from build123d import *

# Parameters (mm, degrees)
EXTRUDE_1_DEPTH      = 5
SKETCH_2_R           = 4
CUT_EXTRUDE_1_DEPTH  = 5
SKETCH_3_R           = 7.5
CUT_EXTRUDE_2_DEPTH  = 10
CUT_EXTRUDE_START    = -10
CUT_EXTRUDE_3_DEPTH  = 10
CUT_EXTRUDE_4_DEPTH  = 10
FILLET_1_R           = 2
SKETCH_6_R           = 6.525
CUT_EXTRUDE_5_DEPTH  = 10
SKETCH_8_R           = 1.5
CUT_EXTRUDE_7_DEPTH  = 10
SKETCH_11_R          = 0.8
CUT_EXTRUDE_8_DEPTH  = 10
SKETCH_13_R          = 1.65
EXTRUDE_3_DEPTH      = 5
FILLET_3_R           = 10
CUT_EXTRUDE_9_DEPTH  = 5
SKETCH_16_W          = 48
SKETCH_16_H          = 16
SKETCH_16_W_2        = 50
CUT_EXTRUDE_10_DEPTH = 2
FILLET_4_SIZE        = 8
SKETCH_17_R          = 12.5
SKETCH_17_R_2        = 12.25
CUT_EXTRUDE_11_DEPTH = 1


with BuildPart() as part:
    # 草图1 → 凸台-拉伸1 (new body)
    with BuildSketch(Plane.XY):
        with BuildLine():
            Line((-30.736828822, 22.472146181), (-0.685809887, 14.645629979))
            ThreePointArc((-0.685809887, 14.645629979), (1.813935823, 14.162064114), (4.35486081, 14))
            Line((4.35486081, 14), (116.18070798, 14))
            ThreePointArc((116.18070798, 14), (120.501201779, 14.472241979), (124.617663724, 15.866666667))
            ThreePointArc((124.617663724, 15.866666667), (149.5, 0), (124.617663724, -15.866666667))
            ThreePointArc((124.617663724, -15.866666667), (120.501201779, -14.472241979), (116.18070798, -14))
            Line((116.18070798, -14), (0, -14))
            ThreePointArc((0, -14), (-4.256709716, -13.337181951), (-8.110358856, -11.411488914))
            Line((-8.110358856, -11.411488914), (-36.971915435, 9.10095979))
            ThreePointArc((-36.971915435, 9.10095979), (-39.424388736, 18.383894386), (-30.736828822, 22.472146181))
        make_face()
    extrude(amount=EXTRUDE_1_DEPTH)

    # 草图2 → 切除-拉伸1 (cut)
    with BuildSketch(Plane.XY.offset(5)):
        with Locations((-32.627080333, 15.214257423)):
            Circle(SKETCH_2_R)
    extrude(amount=-CUT_EXTRUDE_1_DEPTH, mode=Mode.SUBTRACT)

    # 草图3 → 切除-拉伸2 (cut)
    with BuildSketch(Plane.XY.offset(5)):
        Circle(SKETCH_3_R)
    extrude(amount=-CUT_EXTRUDE_2_DEPTH, mode=Mode.SUBTRACT)

    # 草图4 → 切除-拉伸3 (cut)
    with BuildSketch(Plane.XY.offset(5).offset(CUT_EXTRUDE_START)):
        with BuildLine():
            ThreePointArc((-13.498186757, -0.221256097), (-12.235155125, 5.705346533), (-8.506975197, 10.482431635))
            Line((-8.506975197, 10.482431635), (-25.137780404, 14.813774499))
            ThreePointArc((-25.137780404, 14.813774499), (-25.829771931, 12.04462046), (-27.506263415, 9.73454629))
            Line((-27.506263415, 9.73454629), (-13.498186757, -0.221256097))
        make_face()
    extrude(amount=CUT_EXTRUDE_3_DEPTH, mode=Mode.SUBTRACT)

    # 草图5 → 切除-拉伸4 (cut)
    with BuildSketch(Plane.XY.offset(5).offset(CUT_EXTRUDE_START)):
        Polygon((33.945349397, 8), (17.945349397, -8), (33.945349397, -8), align=None)
        with BuildLine():
            ThreePointArc((13.5, 0), (12.826784504, -4.209940534), (10.874281585, -8))
            Line((10.874281585, -8), (26.874281585, 8))
            Line((26.874281585, 8), (10.874281585, 8))
            ThreePointArc((10.874281585, 8), (12.826784504, 4.209940534), (13.5, 0))
        make_face()
        Polygon((54.945349397, -8), (38.945349397, 8), (38.945349397, -8), align=None)
        Polygon((62.016417209, 8), (46.016417209, 8), (62.016417209, -8), align=None)
        Polygon((83.016417209, 8), (67.016417209, 8), (67.016417209, -8), align=None)
        Polygon((90.087485021, 8), (74.087485021, -8), (90.087485021, -8), align=None)
    extrude(amount=CUT_EXTRUDE_4_DEPTH, mode=Mode.SUBTRACT)

    # 圆角1
    fillet_1_edges = [part.edges().sort_by_distance(p)[0] for p in [
        (38.945349397, 8, 2.5),
        (54.945349397, -8, 2.5),
        (38.945349397, -8, 2.5),
        (10.874281585, -8, 2.5),
        (10.874281585, 8, 2.5),
        (26.874281585, 8, 2.5),
        (90.087485021, 8, 2.5),
        (90.087485021, -8, 2.5),
        (74.087485021, -8, 2.5),
        (17.945349397, -8, 2.5),
        (33.945349397, 8, 2.5),
        (33.945349397, -8, 2.5),
        (-27.506263415, 9.73454629, 2.5),
        (-25.137780404, 14.813774499, 2.5),
        (-8.506975197, 10.482431635, 2.5),
        (-13.498186757, -0.221256097, 2.5),
        (67.016417209, -8, 2.5),
        (67.016417209, 8, 2.5),
        (83.016417209, 8, 2.5),
        (62.016417209, -8, 2.5),
        (46.016417209, 8, 2.5),
        (62.016417209, 8, 2.5),
    ]]
    fillet(fillet_1_edges, radius=FILLET_1_R)

    # 草图6 → 切除-拉伸5 (cut)
    with BuildSketch(Plane.XY.offset(5)):
        with Locations((132, 0)):
            Circle(SKETCH_6_R)
    extrude(amount=-CUT_EXTRUDE_5_DEPTH, mode=Mode.SUBTRACT)

    # 草图8 → 切除-拉伸7 (cut)
    with BuildSketch(Plane.XY.offset(5)):
        with Locations((141.5, 0)):
            Circle(SKETCH_8_R)
        with Locations((127.25, -8.227241336)):
            Circle(SKETCH_8_R)
        with Locations((127.25, 8.227241336)):
            Circle(SKETCH_8_R)
    extrude(amount=-CUT_EXTRUDE_7_DEPTH, mode=Mode.SUBTRACT)

    # 草图11 → 切除-拉伸8 (cut)
    with BuildSketch(Plane.XY.offset(5)):
        with Locations((66, -12)):
            Circle(SKETCH_11_R)
        with Locations((112, -12)):
            Circle(SKETCH_11_R)
    extrude(amount=-CUT_EXTRUDE_8_DEPTH, mode=Mode.SUBTRACT)

    # 草图13 → 凸台-拉伸3 (add)
    with BuildSketch(Plane(origin=(0, 0, 0), x_dir=(-1, 0, 0), z_dir=(0, 0, -1))):
        with BuildLine():
            Line((13.852186046, -4.540588259), (-8.101408935, -9.534449379))
            Line((-8.101408935, -9.534449379), (6.922184096, -23.45385613))
            ThreePointArc((6.922184096, -23.45385613), (14, -24.248711306), (16.850543177, -17.721715341))
            Line((16.850543177, -17.721715341), (13.852186046, -4.540588259))
        make_face()
        with Locations((11, -19.052558883)):
            Circle(SKETCH_13_R, mode=Mode.SUBTRACT)
    extrude(amount=-EXTRUDE_3_DEPTH)

    # 圆角3
    fillet_3_edges = [part.edges().sort_by_distance(p)[0] for p in [
        (3.281619098, -14, 2.5),
        (-14.398527657, -6.942369598, 2.5),
    ]]
    fillet(fillet_3_edges, radius=FILLET_3_R)

    # 草图15 → 切除-拉伸9 (cut)
    with BuildSketch(Plane(origin=(0, 0, 0), x_dir=(-1, 0, 0), z_dir=(0, 0, -1))):
        with BuildLine():
            Line((1.631482745, -15.143918385), (4.739694736, -18.023686685))
            ThreePointArc((4.739694736, -18.023686685), (6.449635066, -18.525605556), (7.88116063, -17.464213523))
            ThreePointArc((7.88116063, -17.464213523), (9.25, -16.02146997), (11.183872253, -15.557392078))
            ThreePointArc((11.183872253, -15.557392078), (12.818827499, -14.848350591), (13.239123171, -13.11653939))
            Line((13.239123171, -13.11653939), (12.299276662, -8.984864696))
            ThreePointArc((12.299276662, -8.984864696), (10.858631775, -7.494474843), (8.870653374, -8.081553608))
            ThreePointArc((8.870653374, -8.081553608), (6, -10.392304845), (2.56350404, -11.722987974))
            ThreePointArc((2.56350404, -11.722987974), (1.061089715, -13.151088389), (1.631482745, -15.143918385))
        make_face()
    extrude(amount=-CUT_EXTRUDE_9_DEPTH, mode=Mode.SUBTRACT)

    # 草图16 → 切除-拉伸10 (cut)
    with BuildSketch(Plane(origin=(0, 0, 0), x_dir=(-1, 0, 0), z_dir=(0, 0, -1))):
        with Locations((-84.267784395, 0)):
            Rectangle(SKETCH_16_W, SKETCH_16_H)
        with Locations((-35.267784395, 0)):
            Rectangle(SKETCH_16_W_2, SKETCH_16_H)
    extrude(amount=-CUT_EXTRUDE_10_DEPTH, mode=Mode.SUBTRACT)

    # 圆角4
    # a fillet whose section is not a circle: 8 mm, written as the material it adds along each edge
    with BuildSketch(Plane(origin=(108.267784395, 8, 0), x_dir=(-1, 0, 0), z_dir=(0, 0, 1)), Plane(origin=(108.267784395, -8, 0), x_dir=(0, 1, 0), z_dir=(0, 0, 1))) as fillet_4_piece_1:
        with BuildLine():
            add(Edge.make_bspline([(FILLET_4_SIZE, 0), (FILLET_4_SIZE * 0.831801948466, 0), (FILLET_4_SIZE * 0.663603896932, 0), (FILLET_4_SIZE * 0.292893218813, FILLET_4_SIZE * 0.0716919198361), (FILLET_4_SIZE * 0.0716919198361, FILLET_4_SIZE * 0.292893218813), (0, FILLET_4_SIZE * 0.663603896932), (0, FILLET_4_SIZE * 0.831801948466), (0, FILLET_4_SIZE)], knots=[0, 0, 0, 0, 0, 0, 0.5, 0.5, 1, 1, 1, 1, 1, 1], degree=5))
            Line((0, FILLET_4_SIZE), (0, 0))
            Line((0, 0), (FILLET_4_SIZE, 0))
        make_face()
    extrude(amount=2)
    with BuildSketch(Plane(origin=(10.267784395, -8, 0), x_dir=(0, 1, 0), z_dir=(0, 0, 1))) as fillet_4_piece_2:
        with BuildLine():
            add(Edge.make_bspline([(FILLET_4_SIZE, 0), (FILLET_4_SIZE * 0.831801948466, 0), (FILLET_4_SIZE * 0.663603896932, 0), (FILLET_4_SIZE * 0.292893218813, -FILLET_4_SIZE * 0.0716919198361), (FILLET_4_SIZE * 0.0716919198361, -FILLET_4_SIZE * 0.292893218813), (0, -FILLET_4_SIZE * 0.663603896932), (0, -FILLET_4_SIZE * 0.831801948466), (0, -FILLET_4_SIZE)], knots=[0, 0, 0, 0, 0, 0, 0.5, 0.5, 1, 1, 1, 1, 1, 1], degree=5))
            Line((0, -FILLET_4_SIZE), (0, 0))
            Line((0, 0), (FILLET_4_SIZE, 0))
        make_face()
    extrude(amount=2)
    with BuildSketch(Plane(origin=(10.267784395, 8, 0), x_dir=(0, -1, 0), z_dir=(0, 0, 1))) as fillet_4_piece_3_section:
        with BuildLine():
            add(Edge.make_bspline([(FILLET_4_SIZE, 0), (FILLET_4_SIZE * 0.831801948466, 0), (FILLET_4_SIZE * 0.663603896932, 0), (FILLET_4_SIZE * 0.292893218813, FILLET_4_SIZE * 0.0716919198361), (FILLET_4_SIZE * 0.0716919198361, FILLET_4_SIZE * 0.292893218813), (0, FILLET_4_SIZE * 0.663603896932), (0, FILLET_4_SIZE * 0.831801948466), (0, FILLET_4_SIZE)], knots=[0, 0, 0, 0, 0, 0, 0.5, 0.5, 1, 1, 1, 1, 1, 1], degree=5))
            Line((0, FILLET_4_SIZE), (0, 0))
            Line((0, 0), (FILLET_4_SIZE, 0))
        make_face()
    fillet_4_piece_3 = extrude(amount=22, mode=Mode.PRIVATE)
    fillet_4_piece_3 = split(fillet_4_piece_3, bisect_by=Plane(origin=(10.267784395, 8, 5), z_dir=(0, 0, -1)), keep=Keep.TOP, mode=Mode.PRIVATE)
    add(fillet_4_piece_3)

    # 草图17 → 切除-拉伸11 (cut)
    with BuildSketch(Plane.XY.offset(5)):
        with Locations((132, 0)):
            Circle(SKETCH_17_R)
        Circle(SKETCH_17_R_2)
    extrude(amount=-CUT_EXTRUDE_11_DEPTH, mode=Mode.SUBTRACT)


solid = part.part
Design review of the part built by this model. Coordinates are the model's own, in mm. A direction names the side the tool comes from. Give positions to 0.01 mm unless a question says otherwise; leave off trailing zeros. Write each loop counter-clockwise with the first axis right and the second up, starting at its lowest first coordinate (ties: lowest second). Pieces come first, ordered by that corner, then holes. Notation, with made-up numbers: M 4.25,49.25 L 32.25,49.25 A12 cw 32.25,71.25 Z; hole C 74,-36.5 d5. An arc over 180 degrees is marked long. Answer as a JSON object with one key per item and string values. Group by question number.
1) For line 1 along X through (y, z) = (4.5, 1.4) (3 decimals); line 2 along Y through (x, z) = (132, 4.2); line 3 along Y through (x, z) = (48.5, 0.75), list the stretches that pass through material, from the lowest coordinate up.
2) We need section A-A (x = 132). Give the boundary of the cut face in (y, z) (3 decimals), and give its area (3 significant figures).
3) Tool access review of faces 1 (the face through (143.923, 3.755, 4.507)), 2 (the face through (59, 8, 1)), 3 (the face through (-15.922, 18.614, 2.465)), 4 (the face through (82.15, 0.06, 3.48)), 5 (the face through (62, 10, 0)): name each direction out of +Z, -Z, +X, -X, +Y, -Y from which nothing blocks a thin tool from reaching the whole face with its end or side.
4) Clearance check with flat-ended pins moving along their axes: pin 1 Ø1.8 at (x, y) = (66, -12) entering from +Z; pin 2 Ø2.5 at (x, z) = (39, 3.5) entering from +Y; pin 3 Ø1.5 at (y, z) = (1, 2) entering from +X; pin 4 Ø1.5 at (x, z) = (61, 3) entering from -Y. State where each tip first meets the part, or that it passes through.
5) Mouldability with a two-part tool opening along Y and no side actions: class faces 6 (the face through (-12.776, -11.08, 2.465)), 7 (the face through (1.779, 14.167, 2.465)), 8 (the face through (-39.485, 18.251, 2.465)) as released by +Y, released by -Y, zero draft, split by the parting line, or undercut.
6) We need section C-C (z = 0.9). Count the separate pieces of the cut face and the enclosed holes in it, and give its area (3 significant figures).
7) We need section B-B (x = 75). Give the boundary of the cut face in (y, z).
Answer key:
{
 "1": {"line 1": "x = -30.498 to -20.141, -12.728 to -6, 6 to 10.898, 107.638 to 127.275, 136.725 to 148.912", "line 2": "y = -17.5 to -12.5, 12.5 to 17.5", "line 3": "y = -14 to -8, 8 to 14"},
 "2": {"outline": "M -17.5,0 L -6.525,0 L -6.525,4 L -12.5,4 L -12.5,5 L -17.5,5 Z; M 6.525,0 L 17.5,0 L 17.5,5 L 12.5,5 L 12.5,4 L 6.525,4 Z", "area": "97.8 mm²"},
 "3": {"face 1": "+Z", "face 2": "-Z", "face 3": "+Z, -Z, +Y", "face 4": "+Z, -Z", "face 5": "-Z, +X, -X, +Y, -Y"},
 "4": {"pin 1": "stops at z = 5", "pin 2": "stops at y = 14", "pin 3": "stops at x = 149.5", "pin 4": "stops at y = -14"},
 "5": {"face 6": "undercut", "face 7": "released by +Y", "face 8": "split by the parting line"},
 "6": {"separate pieces": "1", "enclosed holes": "12", "area": "3,170 mm²"},
 "7": {"outline": "M -14,0 L -8,0 L -8,2 L -0.02,2 L -0.02,5 L -14,5 Z; M 8,0 L 14,0 L 14,5 L 8,5 Z"}
}
